Geometry: final body of the model. Coordinates: model frame, mm. Face numbers are marked on the shaded views. Give positions to 0.01 mm unless a question says otherwise; leave off trailing zeros. Write each loop counter-clockwise with the first axis right and the second up, starting at its lowest first coordinate (ties: lowest second). Pieces come first, ordered by that corner, then holes. Notation, with made-up numbers: (76, -7) -> (133, -7) arc R19 cw to (133, 10) -> close; hole circle Ø9 at (32.5, 29.25). An arc over 180 degrees is marked (long way). Answer as a JSON object with one key per item and string values.
from build123d import *

# Parameters (mm, degrees)
F0_R     = 3.81
F1_DEPTH = 12.7
F3_DEPTH = 25.4
F4_R     = 1.778
F5_DEPTH = 25.4
F7_DEPTH = 0.3175


with BuildPart() as f1:
    # F0 (on Right) → F1 (new body, symmetric)
    with BuildSketch(Plane.YZ):
        Circle(F0_R)
    extrude(amount=F1_DEPTH, both=True)

    # F2 (on face) → F3 (cut)
    with BuildSketch(Plane.YZ.offset(12.7)):
        with BuildLine():
            ThreePointArc((3.6720354029, 1.016), (0, 3.81), (-3.6720354029, 1.016))
            Line((-3.6720354029, 1.016), (3.6720354029, 1.016))
        make_face()
    extrude(amount=-F3_DEPTH, mode=Mode.SUBTRACT)

    # F4 (on face) → F5 (cut)
    with BuildSketch(Plane.XY.offset(1.016)):
        with Locations((-9.7155, 0)):
            Circle(F4_R)
        with Locations((9.7155, 0)):
            Circle(F4_R)
    extrude(amount=-F5_DEPTH, mode=Mode.SUBTRACT)

    # F6 (on face) → F7 (cut)
    with BuildSketch(Plane.XY.offset(1.016)):
        with BuildLine():
            Line((-4.4995615003, 1.651), (4.3904384997, 1.651))
            ThreePointArc((4.3904384997, 1.651), (4.6149449027, 1.743993597), (4.7079384997, 1.9685))
            Line((4.7079384997, 1.9685), (4.7079384997, 2.6035))
            ThreePointArc((4.7079384997, 2.6035), (4.6149449027, 2.828006403), (4.3904384997, 2.921))
            Line((4.3904384997, 2.921), (-4.4995615003, 2.921))
            ThreePointArc((-4.4995615003, 2.921), (-4.7240679033, 2.828006403), (-4.8170615003, 2.6035))
            Line((-4.8170615003, 2.6035), (-4.8170615003, 1.9685))
            ThreePointArc((-4.8170615003, 1.9685), (-4.7240679033, 1.743993597), (-4.4995615003, 1.651))
        make_face()
        with BuildLine():
            ThreePointArc((4.7625, 0.3175), (4.669506403, 0.542006403), (4.445, 0.635))
            Line((4.445, 0.635), (-4.445, 0.635))
            ThreePointArc((-4.445, 0.635), (-4.669506403, 0.542006403), (-4.7625, 0.3175))
            Line((-4.7625, 0.3175), (-4.7625, -0.3175))
            ThreePointArc((-4.7625, -0.3175), (-4.669506403, -0.542006403), (-4.445, -0.635))
            Line((-4.445, -0.635), (4.445, -0.635))
            ThreePointArc((4.445, -0.635), (4.669506403, -0.542006403), (4.7625, -0.3175))
            Line((4.7625, -0.3175), (4.7625, 0.3175))
        make_face()
        with BuildLine():
            ThreePointArc((4.7079384997, -1.9685), (4.6149449027, -1.743993597), (4.3904384997, -1.651))
            Line((4.3904384997, -1.651), (-4.4995615003, -1.651))
            ThreePointArc((-4.4995615003, -1.651), (-4.7240679033, -1.743993597), (-4.8170615003, -1.9685))
            Line((-4.8170615003, -1.9685), (-4.8170615003, -2.6035))
            ThreePointArc((-4.8170615003, -2.6035), (-4.7240679033, -2.828006403), (-4.4995615003, -2.921))
            Line((-4.4995615003, -2.921), (4.3904384997, -2.921))
            ThreePointArc((4.3904384997, -2.921), (4.6149449027, -2.828006403), (4.7079384997, -2.6035))
            Line((4.7079384997, -2.6035), (4.7079384997, -1.9685))
        make_face()
    extrude(amount=-F7_DEPTH, mode=Mode.SUBTRACT)


solid = f1.part
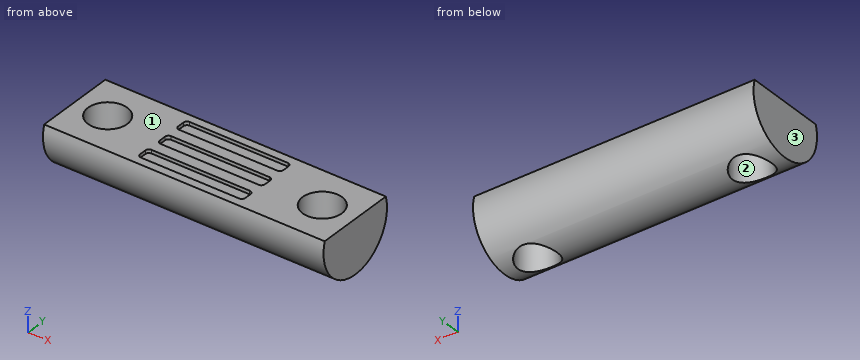
Q1. Cut plane D-D (x = 10.5). Return the cut outline in (y, z).
Values:
{"outline": "(-3.67, 1.02) arc R3.81 ccw to (-1.6, -3.46) -> (-1.6, 1.02) -> close; (1.6, -3.46) arc R3.81 ccw to (3.67, 1.02) -> (1.6, 1.02) -> close"}
Q2. Mould query, pull axis X, two halves, no side actions, for the marked faces 1, 2 and 3. Classes: pulls with the +X half, pulls with the -X half, needs draft (parallel to the pull), parting line crosses it, or undercut.
Values:
{"face 1": "needs draft", "face 2": "undercut", "face 3": "pulls with the -X half"}
Q3. Cut plane C-C (z = 0). Return the cut outline in (x, y).
Values:
{"outline": "(-12.7, -3.81) -> (12.7, -3.81) -> (12.7, 3.81) -> (-12.7, 3.81) -> close; hole circle Ø3.56 at (-9.72, 0); hole circle Ø3.56 at (9.72, 0)"}
Q4. First-contact query: P1, Ø0.6, axis at x = 1.5, y = 2.5, coming from the +Z side; P2, Ø3, axis at x = 9.72, y = 0, coming from the -Z side; P3, Ø2, axis at x = 4.5, y = 1.5, coming from the -Z side. Flat tips, straight axial feed; report the tip coordinate or a pass-through.
Values:
{"P1": "z = 0.7", "P2": "through", "P3": "z = -3.78"}
Q5. Material intervals for L1, parallel to X at y = 0, z = -0.9; L2, parallel to Y at x = -2.75, z = 0.85 (3 decimals); L3, parallel to X at y = -0.75, z = -0.6, sorted ascending. Write a range as from..to.
Values:
{"L1": "-12.7..-11.49, -7.94..7.94, 11.49..12.7", "L2": "-3.714..-2.921, -1.651..-0.635, 0.635..1.651, 2.921..3.714", "L3": "-12.7..-11.33, -8.1..8.1, 11.33..12.7"}
Q6. Cut plane A-A (y = 0). Return the cut outline in (x, z), and give its area (3 significant figures).
Values:
{"outline": "(-12.7, -3.81) -> (-11.49, -3.81) -> (-11.49, 1.02) -> (-12.7, 1.02) -> close; (-7.94, -3.81) -> (7.94, -3.81) -> (7.94, 1.02) -> (4.76, 1.02) -> (4.76, 0.7) -> (-4.76, 0.7) -> (-4.76, 1.02) -> (-7.94, 1.02) -> close; (11.49, -3.81) -> (12.7, -3.81) -> (12.7, 1.02) -> (11.49, 1.02) -> close", "area": "85.2 mm²"}
